Can you work these out from the model? Positions are in its coordinate system, mm. A direction names the side the tool comes from. Give positions to 0.01 mm unless a question says otherwise; leave off trailing zeros. Write each loop counter-clockwise with the first axis right and the second up, starting at its lowest first coordinate (ties: lowest second). Pieces come first, ordered by that corner, then holes. Notation, with made-up numbers: M 29.25,-27.5 L 80.25,-27.5 A30 cw 80.25,0.5 Z; hole C -12,-39 d4. An arc over 180 degrees is marked long. Answer as CSV lines item,"result". Start each with the question number.
```python
from build123d import *

# Parameters (mm, degrees)
F1_DEPTH = 6
F3_DEPTH = 40
F5_DEPTH = 6


with BuildPart() as f1:
    # F0 (on Front) → F1 (new body)
    with BuildSketch(Plane.XZ):
        Polygon((-15, 200), (0, 0), (100, 0), (100, 200), align=None)
        Polygon((100, 200), (100, 0), (200, 0), (215, 200), align=None)
        Polygon((100, 280), (100, 200), (215, 200), align=None)
        Polygon((100, 280), (-15, 200), (100, 200), align=None)
    extrude(amount=F1_DEPTH)

    # F2 (on face) → F3 (join)
    with BuildSketch(Plane.XZ.offset(6)):
        Polygon((100, 280), (-15, 200), (0, 0), (200, 0), (215, 200), align=None)
        Polygon((-8.760511823, 197.0315087877), (100, 272.6909952733), (208.760511823, 197.0315087877), (194.433148664, 6), (5.566851336, 6), align=None, mode=Mode.SUBTRACT)
    extrude(amount=F3_DEPTH)

    # F4 (on face) → F5 (join)
    with BuildSketch(Plane.XZ.offset(46)):
        Polygon((197.733148664, 50), (2.266851336, 50), (5.566851336, 6), (194.433148664, 6), align=None)
        Polygon((2.266851336, 50), (-3.75, 50), (0, 0), (200, 0), (203.75, 50), (197.733148664, 50), (194.433148664, 6), (5.566851336, 6), align=None)
    extrude(amount=F5_DEPTH)


solid = f1.part
```
1) I want a section at C-C, the plane x = 90.5. Please give me the cut outline in (y, z).
2) I want a section at B-B, the plane z = 125. Please give me the cut outline in (x, y) (3 decimals), then the cut area to 3 significant figures.
3) I want a section at A-A, the plane y = -43. Please give me the cut outline in (x, z).
4) Thinking about a two-plate mould opening in X: for faces 5 (the flat face through (153.62, -25.72, 235.39)), 6 (the flat face through (-7.605, -25.636, 101.4)), 7 (the flat face through (99, -52, 25)), 8 (the flat face through (-1.5, -25.7, 100.2)), which applies, released by +X, released by -X, zero draft, split by the parting line, or undercut?
5) I want a section at D-D, the plane z = 179. Please give me the cut outline in (x, y) (3 decimals), then the cut area to 3 significant figures.
6) I'm going to push flat-ended pins straight in: P1, Ø1, axis at x = 47.5, z = 74.5, coming from the -Y side; P2, Ø1, axis at y = -18, z = 120.5, coming from the -X side (3 decimals); P3, Ø4, axis at x = 140.5, y = -46.5, coming from the +Z side. Where does each tip first touch, or does it pass through?
7) On a 3-axis mill with a long thin cutter (end or side, diameter ignored), from which of +Z, -Z, +X, -X, +Y, -Y can I reach the whole of each face in a straight line? I mean faces 1 (the flat face through (101, -26, 6)), 2 (the flat face through (101, -49, 50)), 3 (the flat face through (44.858, -25.72, 234.332)), 4 (the flat face through (99, -26, 0)). Say none if no direction works.
8) I need wall thicknesses on L1, parallel to Y at x = 31, z = 36; L2, parallel to Y at x = 176, z = 122; L3, parallel to Z at x = 167, y = -49. Which ranges of each line are inside material? Lowest first, please. Write a range as from..to.
Values found:
1,outline,"M -52,0 L 0,0 L 0,273.39 L -46,273.39 L -46,266.08 L -6,266.08 L -6,6 L -46,6 L -46,50 L -52,50 Z"
2,outline,"M -9.375,-46 L -3.358,-46 L -3.358,-6 L 203.358,-6 L 203.358,-46 L 209.375,-46 L 209.375,0 L -9.375,0 Z"
2,area,"1,790 mm²"
3,outline,"M -15,200 L 0,0 L 200,0 L 215,200 L 100,280 Z; hole M -8.76,197.03 L 5.57,6 L 194.43,6 L 208.76,197.03 L 100,272.69 Z"
4,face 5,"undercut"
4,face 6,"released by -X"
4,face 7,"zero draft"
4,face 8,"undercut"
5,outline,"M -13.425,-46 L -7.408,-46 L -7.408,-6 L 207.408,-6 L 207.408,-46 L 213.425,-46 L 213.425,0 L -13.425,0 Z"
5,area,"1,840 mm²"
6,P1,"stops at y = -6"
6,P2,"stops at x = -9.075"
6,P3,"stops at z = 253.17"
7,face 1,"none"
7,face 2,"+Z, +X, -X, -Y"
7,face 3,"-Y"
7,face 4,"-Z, +X, -X, +Y, -Y"
8,L1,"y = -52..-46, -6..0"
8,L2,"y = -6..0"
8,L3,"z = 0..50"
